Study the drawing (mm; zero at the part's minimum x, y, z) and answer. A direction names the side the tool comes from. Give positions to 0.01 mm unless a question says otherwise; leave off trailing zeros. Loops run counter-clockwise (first coordinate to the right, second up) from the corner with the lowest first, then second, coordinate; pieces in that order, holes last. Notation, with made-up numbers: M 14,45 L 23,45 A13 cw 23,62 Z; hole C 24.25,60.5 d9. An arc over 180 degrees is marked long. Use one line per item in the form item = value. Start each with the question number.
1. Each of these flat-tipped pins is pushed along its axis until it touches: pin 1 Ø5 at (x, y) = (4.5, 2.5) entering from -Z; pin 2 Ø1.8 at (y, z) = (4.5, 8) entering from +X; pin 3 Ø4.5 at (y, z) = (11.5, 8) entering from +X; pin 4 Ø2 at (y, z) = (6.5, 8) entering from +X. Where does it stop, or does it pass through?
2. The part is cut by section D-D (z = 2). Write down the section's boundary in (x, y), and give its area (3 significant figures).
3. The part is cut by section C-C (x = 1.5). Write down the section's boundary in (y, z).
4. The part is cut by section A-A (z = 8). Write down the section's boundary in (x, y).
5. The part is cut by section B-B (y = 4.5). Write down the section's boundary in (x, z), and give its area (4 significant figures).
6. For the marked faces 5, 6 and 7, determine the directions among +Z, -Z, +X, -X, +Y, -Y from which every point of the face is accessible in a straight line to the end or side of a thin tool.
7. Straight lines are drawn through the part: line 1 (Y direction, x = 8, z = 2.75); line 2 (Y direction, x = 4.6, z = 8); line 3 (X direction, y = 3.75, z = 11.75). For each, find the intervals that lie inside material, in ascending order. Write a range as from..to.
8. The mould has two halves that part along Y. Classify the marked faces 1, 2, 3 and 4: released by +Y, released by -Y, zero draft, split by the parting line, or undercut.
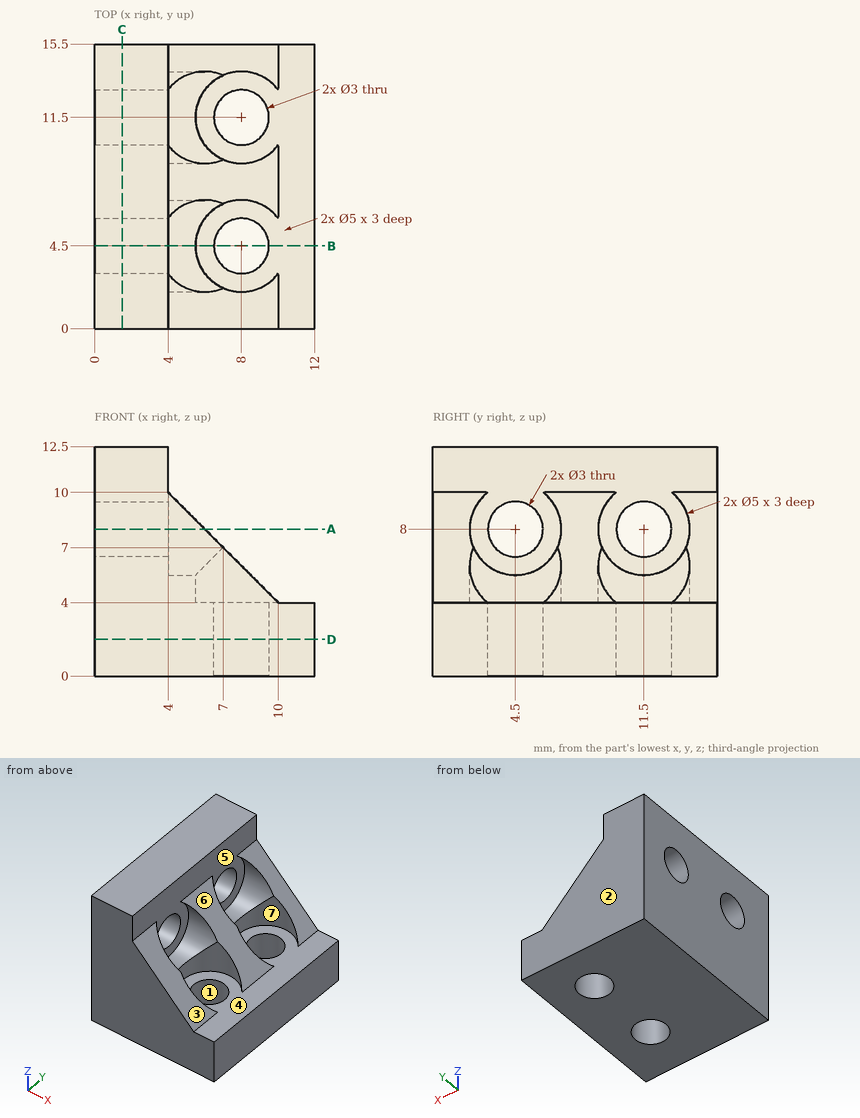
Derived:
q1.pin_1 = 0
q1.pin_2 = through
q1.pin_3 = 4
q1.pin_4 = 6.95
q2.outline = M 0,0 L 12,0 L 12,15.5 L 0,15.5 Z; hole C 8,4.5 d3; hole C 8,11.5 d3
q2.area = 172 mm2
q3.outline = M 0,0 L 15.5,0 L 15.5,12.5 L 0,12.5 Z; hole C 4.5,8 d3; hole C 11.5,8 d3
q4.outline = M 0,0 L 6,0 L 6,2 L 4,2 L 4,3 L 0,3 Z; M 0,6 L 4,6 L 4,7 L 6,7 L 6,9 L 4,9 L 4,10 L 0,10 Z; M 0,13 L 4,13 L 4,14 L 6,14 L 6,15.5 L 0,15.5 Z
q5.outline = M 0,0 L 6.5,0 L 6.5,4 L 5.5,4 L 5.5,5.5 L 4,5.5 L 4,6.5 L 0,6.5 Z; M 0,9.5 L 4,9.5 L 4,12.5 L 0,12.5 Z; M 9.5,0 L 12,0 L 12,4 L 9.5,4 Z
q5.area = 60.25 mm2
q6.face_5 = +X
q6.face_6 = +Z, +X, +Y, -Y
q6.face_7 = +Z
q7.line_1 = 0..3, 6..10, 13..15.5
q7.line_2 = 0..2, 7..9, 14..15.5
q7.line_3 = 0..4
q8.face_1 = undercut
q8.face_2 = released by +Y
q8.face_3 = zero draft
q8.face_4 = undercut
